The model under review builds one solid part; all positions refer to its coordinate system, in mm. Face numbers are marked on the shaded views. A direction names the side the tool comes from. Coordinates: 2 decimals unless noted, no trailing zeros. Write each loop counter-clockwise with the first axis right and the second up, starting at its lowest first coordinate (ties: lowest second). Pieces come first, ordered by that corner, then holes.
```python
from build123d import *

# Parameters (mm, degrees)
ESQUISSE1_R        = 3.5
BOSS_EXTRU_1_DEPTH = 15
ESQUISSE2_RX       = 8
ESQUISSE2_RY       = 4.5
ESQUISSE2_R        = 1
BOSS_EXTRU_2_DEPTH = 2
ESQUISSE4_R        = 3.5
BOSS_EXTRU_3_DEPTH = 5


with BuildPart() as part:
    # Esquisse1 → Boss.-Extru.1 (new body)
    with BuildSketch(Plane(origin=(0, 0, 0), x_dir=(1, 0, 0), z_dir=(0, 1, 0))):
        Circle(ESQUISSE1_R)
    boss_extru_1 = extrude(amount=BOSS_EXTRU_1_DEPTH)

    # Esquisse2 → Boss.-Extru.2 (add)
    with BuildSketch(Plane(origin=(0, 15, 0), x_dir=(1, 0, 0), z_dir=(0, 1, 0))):
        with Locations((0, 0)):
            Ellipse(ESQUISSE2_RX, ESQUISSE2_RY)
        with Locations((6, 0)):
            Circle(ESQUISSE2_R, mode=Mode.SUBTRACT)
        with Locations((-6, 0)):
            Circle(ESQUISSE2_R, mode=Mode.SUBTRACT)
    boss_extru_2 = extrude(amount=BOSS_EXTRU_2_DEPTH)

    # Esquisse4 → Boss.-Extru.3 (add)
    with BuildSketch(Plane(origin=(0, 17, 0), x_dir=(1, 0, 0), z_dir=(0, 1, 0))):
        Circle(ESQUISSE4_R)
    boss_extru_3 = extrude(amount=BOSS_EXTRU_3_DEPTH)

    # Symétrie1: Boss.-Extru.1, Boss.-Extru.2, Boss.-Extru.3 across plane
    add(boss_extru_1.mirror(Plane.ZX))
    add(boss_extru_2.mirror(Plane.ZX))
    add(boss_extru_3.mirror(Plane.ZX))


solid = part.part
```
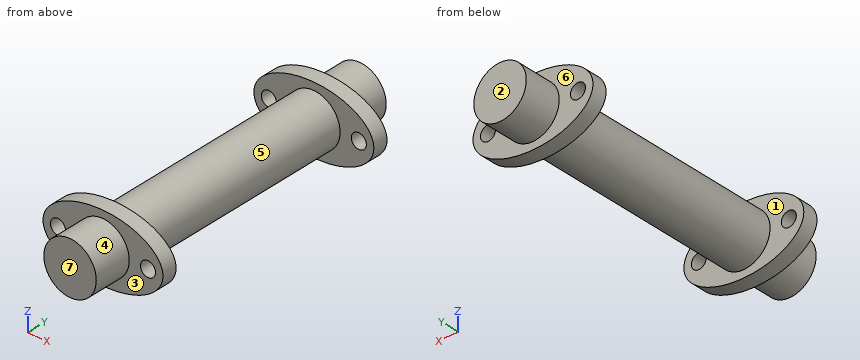
Item 1: For pin 1 (2 mm diameter, centred on y = -6.5, z = 2, fed in from +X); pin 2 (3 mm diameter, centred on x = 1, y = 11, fed in from -Z); pin 3 (2.5 mm diameter, centred on x = 6, z = 0, fed in from +Y), all flat-tipped, find the tip position at first contact; note any pin that passes through.
Solved:
pin 1: stops at x = 3.35
pin 2: stops at z = -3.5
pin 3: stops at y = 17
Item 2: Machinability: for the marked faces 5, 6 and 7, which of the approach directions +Z, -Z, +X, -X, +Y, -Y give a long, thin tool a straight path to every point of the face, cutting with its end or side? Answer none if there is none.
Solved:
face 5: none
face 6: +Y
face 7: +Z, -Z, +X, -X, -Y
Item 3: Take a section at B-B, the plane y = 3. Write out the cut boundary in (x, z).
Solved:
outline: circle Ø7 at (0, 0)
Item 4: Mouldability with a two-part tool opening along Y and no side actions: class the marked faces 1, 2, 3 and 4 as pulls with the +Y half, pulls with the -Y half, needs draft (parallel to the pull), parting line crosses it, or undercut.
Solved:
face 1: undercut
face 2: pulls with the +Y half
face 3: pulls with the -Y half
face 4: needs draft
Item 5: To check wall thickness, follow line 1 along X through (y, z) = (16.15, 0); line 2 along Y through (x, z) = (-4, 1); line 3 along Z through (x, y) = (-6, 16.4). State the ranges of each line that lie inside material, in increasing order.
Solved:
line 1: x = -8 to -7, -5 to 5, 7 to 8
line 2: y = -17 to -15, 15 to 17
line 3: z = -2.98 to -1, 1 to 2.98
Item 6: Take a section at A-A, the plane z = 0. Count the separate pieces of the cut face and the enclosed holes in it, plus the area to 3 significant figures.
Solved:
separate pieces: 5
enclosed holes: 0
area: 328 mm2
